Input: dimensioned drawing with shaded views. Units: mm. Origin: part minimum x, y, z. A direction names the side the tool comes from. Round coordinates to 2 decimals unless told otherwise and drop trailing zeros. Order: outer loops, then holes, each group sorted by start corner. A loop starts at its lowest first (then second) coordinate and runs counter-clockwise, first axis right, second up.
Item 1: Cut plane C-C on y = 8.5. Output: boundary loops of the cut face in (x, z).
Item 2: Cut plane B-B on y = 37. Output: boundary loops of the cut face in (x, z).
Item 3: First-contact query: pin 1 (6 mm diameter, centred on x = 6, y = 27, fed in from -Z); pin 2 (0.7 mm diameter, centred on x = 10, y = 31.5, fed in from -Z); pin 3 (0.7 mm diameter, centred on y = 5, z = 1.5, fed in from -X). Flat tips, straight axial feed; report the tip coordinate or a pass-through.
Item 4: Cut plane A-A on x = 8.5. Output: boundary loops of the cut face in (y, z), then the cut area to 3 significant figures.
Item 5: Mould query, pull axis Z, two halves, no side actions, for the marked faces 1, 2 and 3. Classes: released by +Z, released by -Z, zero draft, split by the parting line, or undercut.
Item 6: Line query: L1, parallel to Y at x = 8.75, z = 5.5; L2, parallel to X at y = 37.5, z = 4.75; L3, parallel to Y at x = 9.5, z = 1. Output: solid intervals per line, ascending.
Item 7: Cut plane D-D on z = 4. Output: boundary loops of the cut face in (x, y), then the cut area to 3 significant figures.
Item 8: Reachability of the marked faces 4, 5 and 6 from +Z, -Z, +X, -X, +Y, -Y: full face, straight path, thin tool, end or side. Return the list, or none.
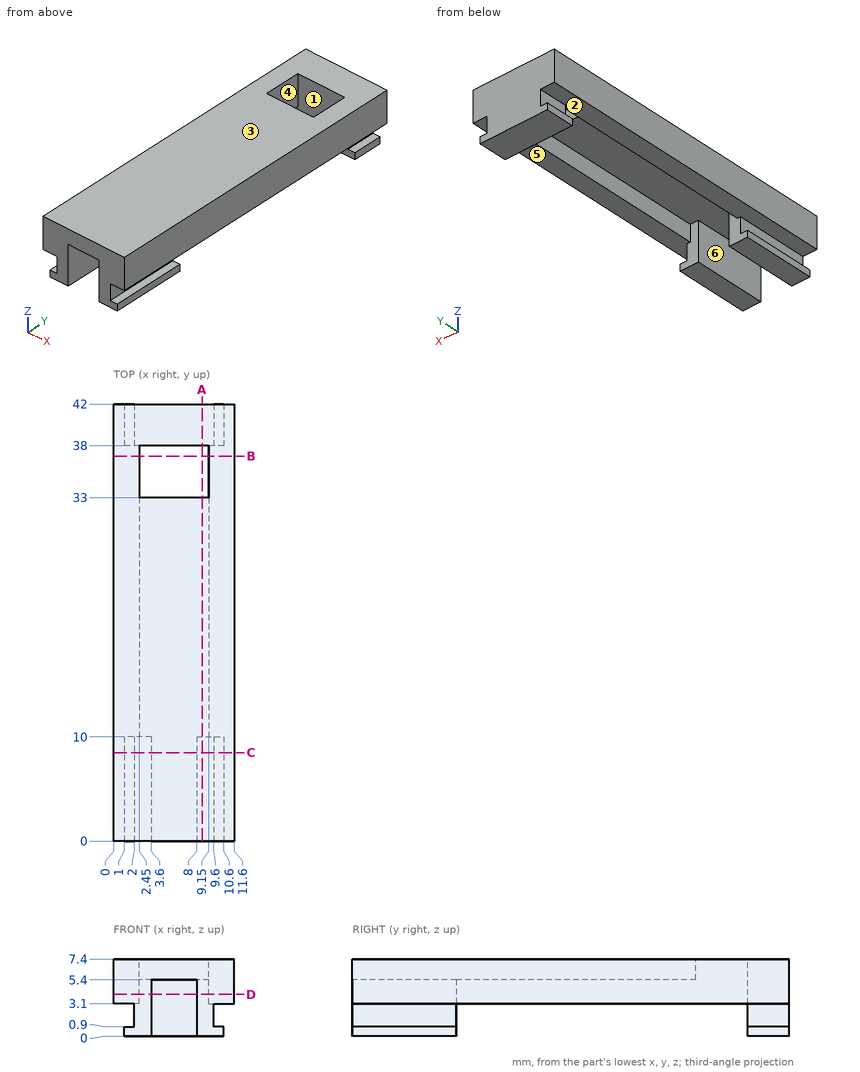
From the geometry:
1. outline: (0, 3.1) - (2, 3.1) - (2, 0.9) - (1, 0.9) - (1, 0) - (3.6, 0) - (3.6, 5.4) - (8, 5.4) - (8, 0) - (10.6, 0) - (10.6, 0.9) - (9.6, 0.9) - (9.6, 3.1) - (11.6, 3.1) - (11.6, 7.4) - (0, 7.4) - close
2. outline: (0, 3.1) - (2.45, 3.1) - (2.45, 7.4) - (0, 7.4) - close; (9.15, 3.1) - (11.6, 3.1) - (11.6, 7.4) - (9.15, 7.4) - close
3. pin 1: stops at z = 5.4
3. pin 2: stops at z = 3.1
3. pin 3: stops at x = 2
4. outline: (0, 0) - (10, 0) - (10, 5.4) - (33, 5.4) - (33, 7.4) - (0, 7.4) - close; (38, 0) - (42, 0) - (42, 7.4) - (38, 7.4) - close
4. area: 150 mm2
5. face 1: zero draft
5. face 2: undercut
5. face 3: released by +Z
6. L1: y = 0 to 33, 38 to 42
6. L2: x = 0 to 2.45, 9.15 to 11.6
6. L3: y = 0 to 10, 38 to 42
7. outline: (0, 0) - (3.6, 0) - (3.6, 10) - (2.45, 10) - (2.45, 38) - (9.15, 38) - (9.15, 10) - (8, 10) - (8, 0) - (11.6, 0) - (11.6, 42) - (0, 42) - close
7. area: 256 mm2
8. face 4: -Z
8. face 5: +X
8. face 6: -Z, -Y
